Here's how the part is built. I have some questions about the finished solid (model axes, mm). Coordinates: 2 decimals unless noted, no trailing zeros. Order: outer loops, then holes, each group sorted by start corner. A loop starts at its lowest first (then second) coordinate and runs counter-clockwise, first axis right, second up. Notation, with made-up numbers: (0.25, 74) - (5.25, 74) arc R10 cw to (5.25, 89) - close; hole circle Ø8 at (24.5, -25). An arc over 180 degrees is marked (long way). Answer in a Markdown table with one row per item. Add a question column.
Item 1: Will these pins go through, and if not, where does the flat tip stop? pin 1 Ø1.5 at (y, z) = (145.5, 3) entering from +X; pin 2 Ø1.5 at (y, z) = (-3.5, 1.5) entering from -X; pin 3 Ø2.5 at (x, z) = (-67.5, 3) entering from -Y.
Item 2: If I drill on line 1 along Y through (x, z) = (6, 1.4); line 2 along Y through (x, z) = (41.5, 1); line 3 along Y through (x, z) = (-12, 1.4), over which ranges is the centre line in solid material (lowest first)? Write a range as from..to.
Item 3: I want a section at C-C (z = 3.8). Count the separate pieces of the cut face and the enclosed holes in it, plus the area to 3 significant figures.
Item 4: I want a section at B-B (y = 149). Please give me the cut outline in (x, z), plus the area to 3 significant figures.
Item 5: I want a section at D-D (y = 114). Please give me the cut outline in (x, z).
Item 6: I want a section at A-A (x = 61). Please give me the cut outline in (y, z), plus the area to 3 significant figures.
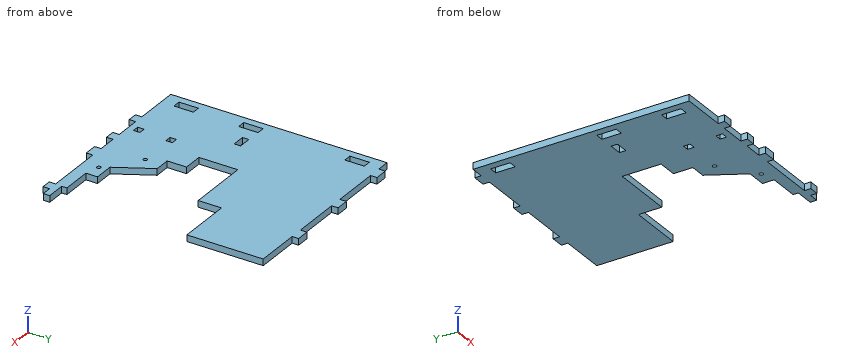
```python
from build123d import *

# Parameters (mm, degrees)
ESQUISSE1_R             = 1.5
BOSS_EXTRU_1_DEPTH      = 5
ESQUISSE2_W             = 6.138933528
ESQUISSE2_H             = 15
ESQUISSE2_W_2           = 5
ESQUISSE2_H_2           = 5
BOSS_EXTRU_2_DEPTH      = 5
ESQUISSE3_W             = 10
ESQUISSE3_H             = 5
BOSS_EXTRU_3_DEPTH      = 5
ESQUISSE4_W             = 10.001975045
ESQUISSE4_H             = 5
ENL_V_MAT_EXTRU_1_DEPTH = 10


with BuildPart() as part:
    # Esquisse1 → Boss.-Extru.1 (new body)
    with BuildSketch(Plane.XY):
        Polygon((0, 0), (37, 0), (37, 18), (27, 18), (12, 45), (0, 45), align=None)
        with Locations((6, 32)):
            Circle(ESQUISSE1_R, mode=Mode.SUBTRACT)
        with Locations((31, 12)):
            Circle(ESQUISSE1_R, mode=Mode.SUBTRACT)
    extrude(amount=BOSS_EXTRU_1_DEPTH)

    # Esquisse2 → Boss.-Extru.2 (add)
    # profile 1 of 2: a face of its own
    with BuildSketch(Plane.XY.offset(5)):
        Polygon((37, 0), (37, 18), (42, 18), (42, 9), (65, 9), (65, 5), (79.5, 5), (79.5, 0), (72, 0), (72, -5), (64.5, -5), (64.5, 0), align=None)
    # profile 2 of 2: a face of its own
    with BuildSketch(Plane.XY.offset(5)):
        Polygon((0, 0), (-5, 0), (-5, -5), (-12.5, -5), (-12.5, 0), (-32.5, 0), (-32.5, -5), (-40, -5), (-40, 0), (-75, 0), (-75, 167), (-65, 167), (-65, 172), (-55, 172), (-55, 167), (30, 167), (30, 172), (40, 172), (40, 167), (75, 167), (75, 108), (33, 108), (33, 90), (-15, 90), (-15, 60), (0, 60), align=None)
        with Locations((-66.228617731, 17.5)):
            Rectangle(ESQUISSE2_W, ESQUISSE2_H, mode=Mode.SUBTRACT)
        with Locations((-66.228617731, 67.5)):
            Rectangle(ESQUISSE2_W, ESQUISSE2_H, mode=Mode.SUBTRACT)
        with Locations((-66.228617731, 149.5)):
            Rectangle(ESQUISSE2_W, ESQUISSE2_H, mode=Mode.SUBTRACT)
        with Locations((-24.5, 7.5)):
            Rectangle(ESQUISSE2_W_2, ESQUISSE2_H_2, mode=Mode.SUBTRACT)
        with Locations((-24.5, 32.5)):
            Rectangle(ESQUISSE2_W_2, ESQUISSE2_H_2, mode=Mode.SUBTRACT)
    extrude(amount=-BOSS_EXTRU_2_DEPTH)

    # Esquisse3 → Boss.-Extru.3 (add)
    with BuildSketch(Plane(origin=(0, 0, 0), x_dir=(-1, 0, 0), z_dir=(0, 0, -1))):
        with Locations((-14.5, -2.5)):
            Rectangle(ESQUISSE3_W, ESQUISSE3_H)
        with Locations((12.893402511, 169.5)):
            Rectangle(ESQUISSE3_W, ESQUISSE3_H)
    extrude(amount=-BOSS_EXTRU_3_DEPTH)

    # Esquisse4 → Enlèv. mat.-Extru.1 (cut)
    with BuildSketch(Plane(origin=(0, 0, 0), x_dir=(-1, 0, 0), z_dir=(0, 0, -1))):
        with Locations((47.271024733, 72.3)):
            Rectangle(ESQUISSE4_W, ESQUISSE4_H)
    extrude(amount=-ENL_V_MAT_EXTRU_1_DEPTH, mode=Mode.SUBTRACT)


solid = part.part
```
Values follow:
| question | item | result |
|---|---|---|
| 1 | pin 1 | stops at x = 75 |
| 1 | pin 2 | stops at x = -40 |
| 1 | pin 3 | stops at y = 0 |
| 2 | line 1 | y = 0..30.5, 33.5..45, 90..167 |
| 2 | line 2 | y = 0..18, 108..167 |
| 2 | line 3 | y = -5..60, 90..172 |
| 3 | separate pieces | 1 |
| 3 | enclosed holes | 8 |
| 3 | area | 18,600 mm^2 |
| 4 | outline | (-75, 0) - (-69.3, 0) - (-69.3, 5) - (-75, 5) - close; (-63.16, 0) - (75, 0) - (75, 5) - (-63.16, 5) - close |
| 4 | area | 719 mm^2 |
| 5 | outline | (-75, 0) - (75, 0) - (75, 5) - (-75, 5) - close |
| 6 | outline | (0, 0) - (9, 0) - (9, 5) - (0, 5) - close; (108, 0) - (167, 0) - (167, 5) - (108, 5) - close |
| 6 | area | 340 mm^2 |
